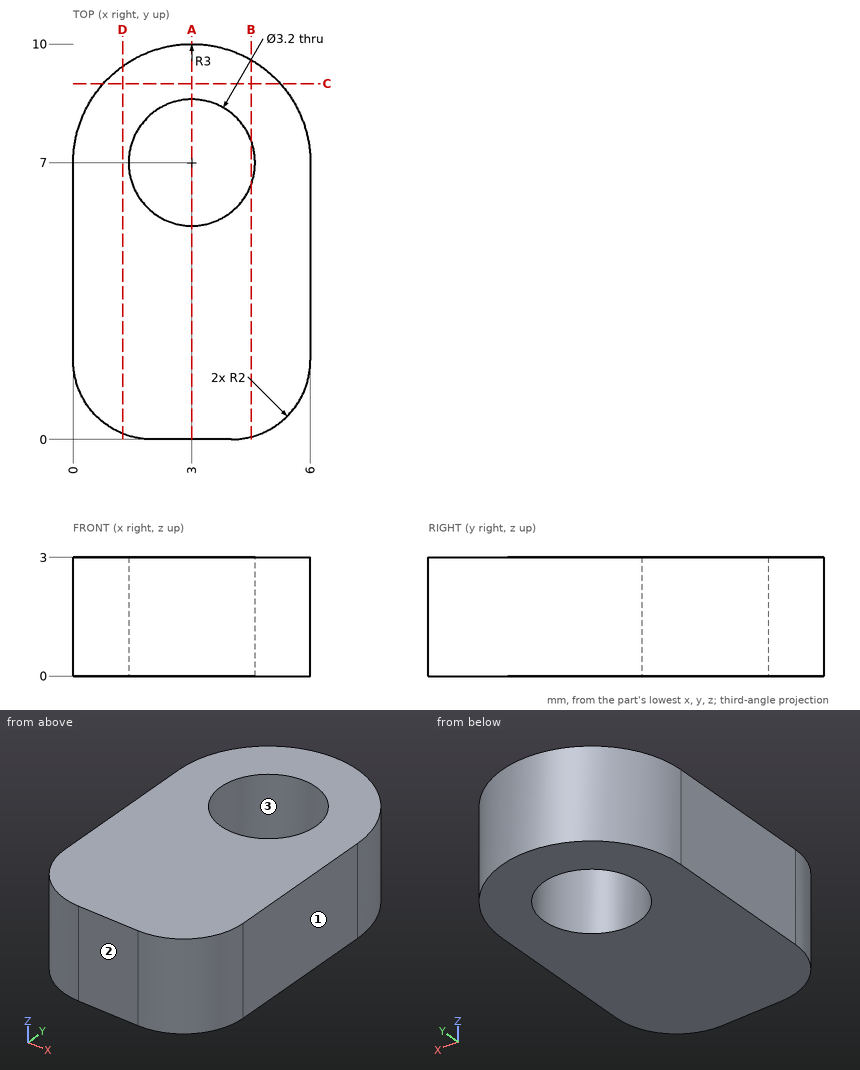
Could you check a few things on this drawing? It's one solid part, dimensions in mm from its lowest x, y, z. Coordinates: 2 decimals unless noted, no trailing zeros. Order: outer loops, then holes, each group sorted by start corner. A loop starts at its lowest first (then second) coordinate and runs counter-clockwise, first axis right, second up. Notation, with made-up numbers: (24, 71.5) - (31, 71.5) arc R21 ccw to (31, 88.5) - close; hole circle Ø6 at (9.5, 0.25). An arc over 180 degrees is marked (long way). Answer as a JSON object with one key per item and string values. Group by question number.
Q1. Imagine slicing it at A-A (x = 3). Please give me the cut outline in (y, z), and give its area (3 significant figures).
Q2. We'd pull the mould along X, two halves only. Please class the marked faces 1, 2 and 3: +X half, -X half, draft (parallel to the pull), parting line (faces both ways), or undercut.
Q3. I need wall thicknesses on line 1 (Y direction, x = 3, z = 0.65); line 2 (X direction, y = 5.75, z = 2.4); line 3 (X direction, y = 7.5, z = 1.45). Which ranges of each line are inside material? Lowest first, please. Write a range as from..to.
Q4. Imagine slicing it at B-B (x = 4.5). Please give me the cut outline in (y, z).
Q5. Will this pin go through, and if not, where does the flat tip stop? P1, Ø3, axis at x = 3, y = 7, coming from the -Z side.
Q6. Imagine slicing it at C-C (y = 9). Please give me the cut outline in (x, z).
Q7. Imagine slicing it at D-D (x = 1.25). Please give me the cut outline in (y, z), and give its area (3 significant figures).
Determined:
{
 "1": {"outline": "(0, 0) - (5.4, 0) - (5.4, 3) - (0, 3) - close; (8.6, 0) - (10, 0) - (10, 3) - (8.6, 3) - close", "area": "20.4 mm2"},
 "2": {"face 1": "+X half", "face 2": "draft", "face 3": "undercut"},
 "3": {"line 1": "y = 0..5.4, 8.6..10", "line 2": "x = 0..2, 4..6", "line 3": "x = 0.04..1.48, 4.52..5.96"},
 "4": {"outline": "(0.06, 0) - (6.44, 0) - (6.44, 3) - (0.06, 3) - close; (7.56, 0) - (9.6, 0) - (9.6, 3) - (7.56, 3) - close"},
 "5": {"P1": "passes through"},
 "6": {"outline": "(0.76, 0) - (5.24, 0) - (5.24, 3) - (0.76, 3) - close"},
 "7": {"outline": "(0.15, 0) - (9.44, 0) - (9.44, 3) - (0.15, 3) - close", "area": "27.9 mm2"}
}
